Check sheet for the modelled part. Datum: model origin and axes. Units: mm. Face numbers are marked on the shaded views. A direction names the side the tool comes from. Round coordinates to 2 decimals unless told otherwise and drop trailing zeros. Write each loop counter-clockwise with the first axis right and the second up, starting at its lowest first coordinate (ties: lowest second). Pieces come first, ordered by that corner, then holes. Notation, with made-up numbers: M -16,87.5 L 28,87.5 A24 cw 28,126.5 Z; hole C 89.5,81 d9. An arc over 180 degrees is marked long. Answer in a Markdown table with one row per item.
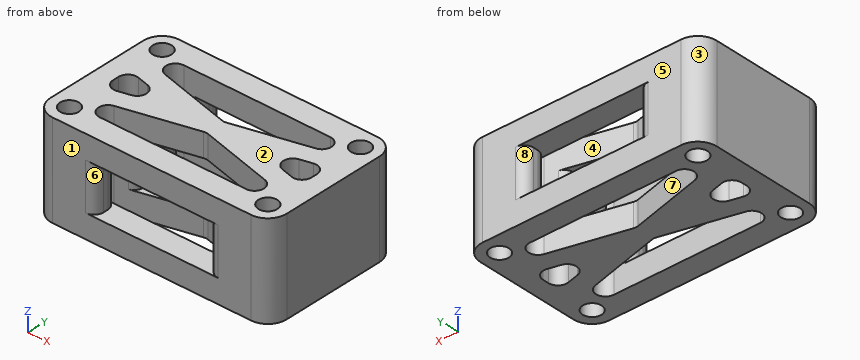
```python
from build123d import *

# Parameters (mm, degrees)
SKETCH_1_W               = 25
SKETCH_1_H               = 15
EXTRUDE_1_DEPTH          = 10
FILLET_4_R               = 2
CUT_EXTRUDE_3_DEPTH      = 10
SKETCH_3_R               = 1
CUT_EXTRUDE_4_DEPTH      = 10
CUT_EXTRUDE_5_DEPTH      = 22.937410968
CUT_EXTRUDE_5_DEPTH_BACK = 22.937410968
SKETCH_4_W               = 12
SKETCH_4_H               = 5
FILLET_5_R               = 1


with BuildPart() as part:
    # 草图1 → 凸台-拉伸1 (new body)
    with BuildSketch(Plane.XY):
        Rectangle(SKETCH_1_W, SKETCH_1_H)
    extrude(amount=EXTRUDE_1_DEPTH)

    # 圆角4
    fillet_4_edges = [part.edges().sort_by_distance(p)[0] for p in [
        (12.5, -7.5, 5),
        (-12.5, -7.5, 5),
        (-12.5, 7.5, 5),
        (12.5, 7.5, 5),
    ]]
    fillet(fillet_4_edges, radius=FILLET_4_R)

    # 草图2 → 切除-拉伸3 (cut)
    with BuildSketch(Plane.XY.offset(10)):
        with BuildLine():
            Line((-0.242535625, -1.091410313), (-7.996324374, -3.0298575))
            ThreePointArc((-7.996324374, -3.0298575), (-8.746296305, -4.122183264), (-7.753788749, -5))
            Line((-7.753788749, -5), (7.753788749, -5))
            ThreePointArc((7.753788749, -5), (8.746296305, -4.122183264), (7.996324374, -3.0298575))
            Line((7.996324374, -3.0298575), (0.242535625, -1.091410313))
            ThreePointArc((0.242535625, -1.091410313), (0, -1.061552813), (-0.242535625, -1.091410313))
        make_face()
        with BuildLine():
            Line((7.753788749, 5), (-7.753788749, 5))
            ThreePointArc((-7.753788749, 5), (-8.746296305, 4.122183264), (-7.996324374, 3.0298575))
            Line((-7.996324374, 3.0298575), (-0.242535625, 1.091410313))
            ThreePointArc((-0.242535625, 1.091410313), (0, 1.061552813), (0.242535625, 1.091410313))
            Line((0.242535625, 1.091410313), (7.996324374, 3.0298575))
            ThreePointArc((7.996324374, 3.0298575), (8.746296305, 4.122183264), (7.753788749, 5))
        make_face()
        with BuildLine():
            Line((-9.257464375, -1.283589687), (-8.003675626, -0.9701425))
            ThreePointArc((-8.003675626, -0.9701425), (-7.246211251, 0), (-8.003675626, 0.9701425))
            Line((-8.003675626, 0.9701425), (-9.257464375, 1.283589687))
            ThreePointArc((-9.257464375, 1.283589687), (-10.115412209, 1.101652625), (-10.5, 0.313447187))
            Line((-10.5, 0.313447187), (-10.5, -0.313447187))
            ThreePointArc((-10.5, -0.313447187), (-10.115412209, -1.101652625), (-9.257464375, -1.283589687))
        make_face()
        with BuildLine():
            Line((10.5, 0.313447187), (10.5, -0.313447187))
            ThreePointArc((10.5, -0.313447187), (10.115412209, -1.101652625), (9.257464375, -1.283589687))
            Line((9.257464375, -1.283589687), (8.003675626, -0.9701425))
            ThreePointArc((8.003675626, -0.9701425), (7.246211251, 0), (8.003675626, 0.9701425))
            Line((8.003675626, 0.9701425), (9.257464375, 1.283589687))
            ThreePointArc((9.257464375, 1.283589687), (10.115412209, 1.101652625), (10.5, 0.313447187))
        make_face()
    extrude(amount=-CUT_EXTRUDE_3_DEPTH, mode=Mode.SUBTRACT)

    # 草图3 → 切除-拉伸4 (cut)
    with BuildSketch(Plane.XY.offset(10)):
        with Locations((-10.5, 5.5)):
            Circle(SKETCH_3_R)
        with Locations(Location((10.5, 5.5, 0), (0, 0, 180))):
            Circle(SKETCH_3_R)
        with Locations((10.5, -5.5)):
            Circle(SKETCH_3_R)
        with Locations(Location((-10.5, -5.5, 0), (0, 0, 180))):
            Circle(SKETCH_3_R)
    extrude(amount=-CUT_EXTRUDE_4_DEPTH, mode=Mode.SUBTRACT)

    # 草图4 → 切除-拉伸5 (cut, two sides: drawn at the far end of the back side and taken through both)
    with BuildSketch(Plane(origin=(0, 7.5, 0), x_dir=(1, 0, 0), z_dir=(0, 1, 0)).offset(-CUT_EXTRUDE_5_DEPTH_BACK)):
        with Locations((0, -5)):
            Rectangle(SKETCH_4_W, SKETCH_4_H)
    extrude(amount=CUT_EXTRUDE_5_DEPTH + CUT_EXTRUDE_5_DEPTH_BACK, mode=Mode.SUBTRACT)

    # 圆角5
    fillet_5_edges = [part.edges().sort_by_distance(p)[0] for p in [
        (6, 2.530776406, 5),
        (-6, 5, 5),
        (-6, 7.5, 5),
        (-6, -5, 5),
        (-6, -7.5, 5),
        (-6, -2.530776406, 5),
        (-6, 2.530776406, 5),
        (6, 7.5, 5),
        (6, 5, 5),
        (6, -2.530776406, 5),
        (6, -5, 5),
        (6, -7.5, 5),
    ]]
    fillet(fillet_5_edges, radius=FILLET_5_R)


solid = part.part
```
1. Go/stop test with flat-tipped pins: pin 1 (3 mm diameter, centred on x = 10.5, y = 5.5, fed in from -Z); pin 2 (1 mm diameter, centred on x = 2, y = -2.5, fed in from -Z). Record where each tip stops, or that it passes through.
Found:
| item | result |
|---|---|
| pin 1 | stops at z = 0 |
| pin 2 | passes through |
2. Access from +Z, -Z, +X, -X, +Y, -Y to the whole of each face (thin tool, end or side, straight path). Record for the marked faces 5, 6, 7 and 8.
Found:
| item | result |
|---|---|
| face 5 | +Z, -Z, +X, -X, +Y |
| face 6 | -Y |
| face 7 | +Z, -Z |
| face 8 | +Y |
3. Scan lines: L1, parallel to X at y = 0, z = 4.5; L2, parallel to Z at x = -3, y = 5.5; L3, parallel to Y at x = 7, z = 8.5. Record each from-to range of solid material in increasing order.
Found:
| item | result |
|---|---|
| L1 | x = -12.5 to -10.5, -7.25 to -6, 6 to 7.25, 10.5 to 12.5 |
| L2 | z = 0 to 2.5, 7.5 to 10 |
| L3 | y = -7.5 to -5, -2.78 to 2.78, 5 to 7.5 |
4. Section check B-B, the plane z = 2.75. Count the separate pieces of the cut face and the enclosed holes in it, and give its area (3 significant figures).
Found:
| item | result |
|---|---|
| separate pieces | 2 |
| enclosed holes | 6 |
| area | 141 mm2 |
5. Section check D-D, the plane x = 7.5. Record the cut outline in (y, z).
Found:
| item | result |
|---|---|
| outline | M -7.5,0 L -5,0 L -5,10 L -7.5,10 Z; M -2.91,0 L -0.67,0 L -0.67,10 L -2.91,10 Z; M 0.67,0 L 2.91,0 L 2.91,10 L 0.67,10 Z; M 5,0 L 7.5,0 L 7.5,10 L 5,10 Z |
6. Draft check along Y on the marked faces 1, 2, 3 and 4. Enter one of: +Y half, -Y half, draft (parallel to the pull), parting line (faces both ways), or undercut.
Found:
| item | result |
|---|---|
| face 1 | -Y half |
| face 2 | draft |
| face 3 | +Y half |
| face 4 | undercut |
7. Section check A-A, the plane y = 4. Record the cut outline in (x, z), and give its area (3 significant figures).
Found:
| item | result |
|---|---|
| outline | M -12.5,0 L -8.75,0 L -8.75,10 L -12.5,10 Z; M 8.75,0 L 12.5,0 L 12.5,10 L 8.75,10 Z |
| area | 74.9 mm2 |
8. Section check C-C, the plane x = 2.75. Record the cut outline in (y, z).
Found:
| item | result |
|---|---|
| outline | M -7.5,0 L -5,0 L -5,2.5 L -7.5,2.5 Z; M -7.5,7.5 L -5,7.5 L -5,10 L -7.5,10 Z; M -1.72,0 L 1.72,0 L 1.72,2.5 L -1.72,2.5 Z; M -1.72,7.5 L 1.72,7.5 L 1.72,10 L -1.72,10 Z; M 5,0 L 7.5,0 L 7.5,2.5 L 5,2.5 Z; M 5,7.5 L 7.5,7.5 L 7.5,10 L 5,10 Z |
